Source: CAD feature listing. Evaluate the final solid. Frame: model axes, mm. A direction names the side the tool comes from. Round coordinates to 2 decimals unless told otherwise and drop trailing zeros.
Item 1: Access query for faces 4 (the flat face through (-1478, 345.908, 1)), 5 (the flat face through (-1481, 338.408, 1)), 6 (the flat face through (-1394, 368.908, 1)). Directions: +Z, -Z, +X, -X, +Y, -Y. A direction counts if a zero-diameter tool reaches every point of the face in a straight line with its end or side. Return the directions, or none.
Item 2: Ray query, L1, parallel to Y at x = -1445, z = 2.55; L2, parallel to Y at x = -1467.5, z = 2.3; L3, parallel to X at y = 367, z = 2.4. Return the intervals inside material, ascending.
Item 3: Section query A-A on z = 1.35. Give the number of separate pieces and of enclosed holes in the cut face, then the cut area to 3 significant figures.
Item 4: First-contact query: P1, Ø4, axis at x = -1446.73, y = 365.41, coming from the +Z side; P2, Ø2.5, axis at x = -1446.73, y = 356.41, coming from the +Z side. Flat tips, straight axial feed; report the tip coordinate or a pass-through.
Item 5: Pull-direction query (Y, two-part tool) for faces 1 (the flat face through (-1388, 363.908, 1)), 2 (the flat face through (-1383.727, 342, 1)), 3 (the flat face through (-1433, 378.908, 1)); classes: released by +Y, released by -Y, zero draft, split by the parting line, or undercut.
```python
from build123d import *

# Parameters (mm, degrees)
MODEL_R                 = 1.5
SALIENTE_EXTRUIR1_DEPTH = 3


with BuildPart() as part:
    # Model → Saliente-Extruir1 (new body)
    with BuildSketch(Plane.XY):
        with BuildLine():
            Line((-1383.726934946, 374.408179756), (-1386.726934946, 374.408179756))
            Line((-1386.726934946, 374.408179756), (-1386.726934946, 378.908179756))
            Line((-1386.726934946, 378.908179756), (-1479.726934946, 378.908179756))
            Line((-1479.726934946, 378.908179756), (-1479.726934946, 374.408179756))
            Line((-1479.726934946, 374.408179756), (-1482.726934946, 374.408179756))
            Line((-1482.726934946, 374.408179756), (-1482.726934946, 366.908179756))
            Line((-1482.726934946, 366.908179756), (-1473.851934946, 366.908179756))
            Line((-1473.851934946, 366.908179756), (-1473.851934946, 368.158179756))
            ThreePointArc((-1473.851934946, 368.158179756), (-1473.632265032, 368.688509842), (-1473.101934946, 368.908179756))
            Line((-1473.101934946, 368.908179756), (-1471.351934946, 368.908179756))
            ThreePointArc((-1471.351934946, 368.908179756), (-1470.82160486, 368.688509842), (-1470.601934946, 368.158179756))
            Line((-1470.601934946, 368.158179756), (-1470.601934946, 366.908179756))
            Line((-1470.601934946, 366.908179756), (-1466.976934946, 366.908179756))
            ThreePointArc((-1466.976934946, 366.908179756), (-1466.44660486, 366.688509842), (-1466.226934946, 366.158179756))
            Line((-1466.226934946, 366.158179756), (-1466.226934946, 364.658179756))
            ThreePointArc((-1466.226934946, 364.658179756), (-1466.44660486, 364.127849671), (-1466.976934946, 363.908179756))
            Line((-1466.976934946, 363.908179756), (-1470.601934946, 363.908179756))
            Line((-1470.601934946, 363.908179756), (-1470.601934946, 362.658179756))
            ThreePointArc((-1470.601934946, 362.658179756), (-1470.82160486, 362.127849671), (-1471.351934946, 361.908179756))
            Line((-1471.351934946, 361.908179756), (-1473.101934946, 361.908179756))
            ThreePointArc((-1473.101934946, 361.908179756), (-1473.632265032, 362.127849671), (-1473.851934946, 362.658179756))
            Line((-1473.851934946, 362.658179756), (-1473.851934946, 363.908179756))
            Line((-1473.851934946, 363.908179756), (-1482.726934946, 363.908179756))
            Line((-1482.726934946, 363.908179756), (-1482.726934946, 348.908179756))
            Line((-1482.726934946, 348.908179756), (-1473.851934946, 348.908179756))
            Line((-1473.851934946, 348.908179756), (-1473.851934946, 350.158179756))
            ThreePointArc((-1473.851934946, 350.158179756), (-1473.632265032, 350.688509842), (-1473.101934946, 350.908179756))
            Line((-1473.101934946, 350.908179756), (-1471.351934946, 350.908179756))
            ThreePointArc((-1471.351934946, 350.908179756), (-1470.82160486, 350.688509842), (-1470.601934946, 350.158179756))
            Line((-1470.601934946, 350.158179756), (-1470.601934946, 348.908179756))
            Line((-1470.601934946, 348.908179756), (-1466.976934946, 348.908179756))
            ThreePointArc((-1466.976934946, 348.908179756), (-1466.44660486, 348.688509842), (-1466.226934946, 348.158179756))
            Line((-1466.226934946, 348.158179756), (-1466.226934946, 346.658179756))
            ThreePointArc((-1466.226934946, 346.658179756), (-1466.44660486, 346.127849671), (-1466.976934946, 345.908179756))
            Line((-1466.976934946, 345.908179756), (-1470.601934946, 345.908179756))
            Line((-1470.601934946, 345.908179756), (-1470.601934946, 344.658179756))
            ThreePointArc((-1470.601934946, 344.658179756), (-1470.82160486, 344.127849671), (-1471.351934946, 343.908179757))
            Line((-1471.351934946, 343.908179757), (-1473.101934946, 343.908179757))
            ThreePointArc((-1473.101934946, 343.908179757), (-1473.632265032, 344.127849671), (-1473.851934946, 344.658179756))
            Line((-1473.851934946, 344.658179756), (-1473.851934946, 345.908179756))
            Line((-1473.851934946, 345.908179756), (-1482.726934946, 345.908179756))
            Line((-1482.726934946, 345.908179756), (-1482.726934946, 338.408179757))
            Line((-1482.726934946, 338.408179757), (-1479.726934946, 338.408179757))
            Line((-1479.726934946, 338.408179757), (-1479.726934946, 333.908179756))
            Line((-1479.726934946, 333.908179756), (-1386.726934946, 333.908179756))
            Line((-1386.726934946, 333.908179756), (-1386.726934946, 338.408179757))
            Line((-1386.726934946, 338.408179757), (-1383.726934946, 338.408179757))
            Line((-1383.726934946, 338.408179757), (-1383.726934946, 345.908179756))
            Line((-1383.726934946, 345.908179756), (-1392.601934946, 345.908179756))
            Line((-1392.601934946, 345.908179756), (-1392.601934946, 344.658179756))
            ThreePointArc((-1392.601934946, 344.658179756), (-1392.82160486, 344.127849671), (-1393.351934946, 343.908179757))
            Line((-1393.351934946, 343.908179757), (-1395.101934946, 343.908179757))
            ThreePointArc((-1395.101934946, 343.908179757), (-1395.632265032, 344.127849671), (-1395.851934946, 344.658179756))
            Line((-1395.851934946, 344.658179756), (-1395.851934946, 345.908179756))
            Line((-1395.851934946, 345.908179756), (-1399.476934946, 345.908179756))
            ThreePointArc((-1399.476934946, 345.908179756), (-1400.007265032, 346.127849671), (-1400.226934946, 346.658179756))
            Line((-1400.226934946, 346.658179756), (-1400.226934946, 348.158179756))
            ThreePointArc((-1400.226934946, 348.158179756), (-1400.007265032, 348.688509842), (-1399.476934946, 348.908179756))
            Line((-1399.476934946, 348.908179756), (-1395.851934946, 348.908179756))
            Line((-1395.851934946, 348.908179756), (-1395.851934946, 350.158179756))
            ThreePointArc((-1395.851934946, 350.158179756), (-1395.632265032, 350.688509842), (-1395.101934946, 350.908179756))
            Line((-1395.101934946, 350.908179756), (-1393.351934946, 350.908179756))
            ThreePointArc((-1393.351934946, 350.908179756), (-1392.82160486, 350.688509842), (-1392.601934946, 350.158179756))
            Line((-1392.601934946, 350.158179756), (-1392.601934946, 348.908179756))
            Line((-1392.601934946, 348.908179756), (-1383.726934946, 348.908179756))
            Line((-1383.726934946, 348.908179756), (-1383.726934946, 363.908179756))
            Line((-1383.726934946, 363.908179756), (-1392.601934946, 363.908179756))
            Line((-1392.601934946, 363.908179756), (-1392.601934946, 362.658179756))
            ThreePointArc((-1392.601934946, 362.658179756), (-1392.82160486, 362.127849671), (-1393.351934946, 361.908179756))
            Line((-1393.351934946, 361.908179756), (-1395.101934946, 361.908179756))
            ThreePointArc((-1395.101934946, 361.908179756), (-1395.632265032, 362.127849671), (-1395.851934946, 362.658179756))
            Line((-1395.851934946, 362.658179756), (-1395.851934946, 363.908179756))
            Line((-1395.851934946, 363.908179756), (-1399.476934946, 363.908179756))
            ThreePointArc((-1399.476934946, 363.908179756), (-1400.007265032, 364.127849671), (-1400.226934946, 364.658179756))
            Line((-1400.226934946, 364.658179756), (-1400.226934946, 366.158179756))
            ThreePointArc((-1400.226934946, 366.158179756), (-1400.007265032, 366.688509842), (-1399.476934946, 366.908179756))
            Line((-1399.476934946, 366.908179756), (-1395.851934946, 366.908179756))
            Line((-1395.851934946, 366.908179756), (-1395.851934946, 368.158179756))
            ThreePointArc((-1395.851934946, 368.158179756), (-1395.632265032, 368.688509842), (-1395.101934946, 368.908179756))
            Line((-1395.101934946, 368.908179756), (-1393.351934946, 368.908179756))
            ThreePointArc((-1393.351934946, 368.908179756), (-1392.82160486, 368.688509842), (-1392.601934946, 368.158179756))
            Line((-1392.601934946, 368.158179756), (-1392.601934946, 366.908179756))
            Line((-1392.601934946, 366.908179756), (-1383.726934946, 366.908179756))
            Line((-1383.726934946, 366.908179756), (-1383.726934946, 374.408179756))
        make_face()
        with Locations((-1401.727545355, 356.408179756)):
            Circle(MODEL_R, mode=Mode.SUBTRACT)
        with Locations((-1464.727545355, 356.408179756)):
            Circle(MODEL_R, mode=Mode.SUBTRACT)
        with Locations((-1455.727545355, 356.408179756)):
            Circle(MODEL_R, mode=Mode.SUBTRACT)
        with Locations((-1410.727545355, 356.408179756)):
            Circle(MODEL_R, mode=Mode.SUBTRACT)
        with Locations((-1446.727545355, 356.408179756)):
            Circle(MODEL_R, mode=Mode.SUBTRACT)
        with Locations((-1437.727545355, 356.408179756)):
            Circle(MODEL_R, mode=Mode.SUBTRACT)
        with Locations((-1428.727545355, 356.408179756)):
            Circle(MODEL_R, mode=Mode.SUBTRACT)
        with Locations((-1419.727545355, 356.408179756)):
            Circle(MODEL_R, mode=Mode.SUBTRACT)
        with Locations((-1455.727545355, 365.408179756)):
            Circle(MODEL_R, mode=Mode.SUBTRACT)
        with Locations((-1446.727545355, 365.408179756)):
            Circle(MODEL_R, mode=Mode.SUBTRACT)
        with Locations((-1437.727545355, 365.408179756)):
            Circle(MODEL_R, mode=Mode.SUBTRACT)
        with Locations((-1428.727545355, 365.408179756)):
            Circle(MODEL_R, mode=Mode.SUBTRACT)
        with Locations((-1419.727545355, 365.408179756)):
            Circle(MODEL_R, mode=Mode.SUBTRACT)
        with Locations((-1410.727545355, 365.408179756)):
            Circle(MODEL_R, mode=Mode.SUBTRACT)
        with Locations((-1455.727545355, 338.408179757)):
            Circle(MODEL_R, mode=Mode.SUBTRACT)
        with Locations((-1446.727545355, 338.408179757)):
            Circle(MODEL_R, mode=Mode.SUBTRACT)
        with Locations((-1437.727545355, 338.408179757)):
            Circle(MODEL_R, mode=Mode.SUBTRACT)
        with Locations((-1428.727545355, 338.408179757)):
            Circle(MODEL_R, mode=Mode.SUBTRACT)
        with Locations((-1419.727545355, 338.408179757)):
            Circle(MODEL_R, mode=Mode.SUBTRACT)
        with Locations((-1410.727545355, 338.408179757)):
            Circle(MODEL_R, mode=Mode.SUBTRACT)
        with BuildLine():
            Line((-1448.226934946, 350.408179756), (-1418.226934946, 350.408179756))
            ThreePointArc((-1418.226934946, 350.408179756), (-1416.726934946, 348.908179756), (-1418.226934946, 347.408179756))
            Line((-1418.226934946, 347.408179756), (-1448.226934946, 347.408179756))
            ThreePointArc((-1448.226934946, 347.408179756), (-1449.726934946, 348.908179756), (-1448.226934946, 350.408179756))
        make_face(mode=Mode.SUBTRACT)
        with BuildLine():
            Line((-1448.226934946, 374.408179756), (-1418.226934946, 374.408179756))
            ThreePointArc((-1418.226934946, 374.408179756), (-1416.726934946, 372.908179756), (-1418.226934946, 371.408179756))
            Line((-1418.226934946, 371.408179756), (-1448.226934946, 371.408179756))
            ThreePointArc((-1448.226934946, 371.408179756), (-1449.726934946, 372.908179756), (-1448.226934946, 374.408179756))
        make_face(mode=Mode.SUBTRACT)
    extrude(amount=SALIENTE_EXTRUIR1_DEPTH)


solid = part.part
```
Data:
1. face 4: +Z, -Z, -X
1. face 5: +Z, -Z, -X, -Y
1. face 6: +Z, -Z
2. L1: y = 333.91 to 347.41, 350.41 to 371.41, 374.41 to 378.91
2. L2: y = 333.91 to 345.91, 348.91 to 363.91, 366.91 to 378.91
2. L3: x = -1482.73 to -1473.85, -1470.6 to -1395.85, -1392.6 to -1383.73
3. separate pieces: 1
3. enclosed holes: 22
3. area: 3,820 mm2
4. P1: stops at z = 3
4. P2: passes through
5. face 1: undercut
5. face 2: zero draft
5. face 3: released by +Y
